from build123d import *

# Parameters (mm, degrees)
SKETCH1_W           = 177.8
SKETCH1_H           = 355.6
BOSS_EXTRUDE1_DEPTH = 12.7
BOSS_EXTRUDE2_DEPTH = 76.2


with BuildPart() as part:
    # Sketch1 → Boss-Extrude1 (new, symmetric)
    with BuildSketch(Plane(origin=(0, 0, 0), x_dir=(1, 0, 0), z_dir=(0, 1, 0))):
        Rectangle(SKETCH1_W, SKETCH1_H)
    extrude(amount=BOSS_EXTRUDE1_DEPTH, both=True)

    # Sketch2 → Boss-Extrude2 (add, symmetric)
    with BuildSketch(Plane(origin=(0, 0, 0), x_dir=(0, 0, -1), z_dir=(1, 0, 0))):
        with BuildLine():
            Line((-152.4, -12.7), (-152.4, 38.1))
            ThreePointArc((-152.4, 38.1), (-127, 63.5), (-101.6, 38.1))
            Line((-101.6, 38.1), (-101.6, -12.7))
            ThreePointArc((-101.6, -12.7), (-127, -38.1), (-152.4, -12.7))
        make_face()
        with BuildLine():
            Line((101.6, -12.7), (101.6, 38.1))
            ThreePointArc((101.6, 38.1), (127, 63.5), (152.4, 38.1))
            Line((152.4, 38.1), (152.4, -12.7))
            ThreePointArc((152.4, -12.7), (127, -38.1), (101.6, -12.7))
        make_face()
    extrude(amount=BOSS_EXTRUDE2_DEPTH, both=True)


solid = part.part
The model under review builds one solid part; all positions refer to its coordinate system, in mm. A direction names the side the tool comes from. Give positions to 0.01 mm unless a question says otherwise; leave off trailing zeros. Order: outer loops, then holes, each group sorted by start corner. A loop starts at its lowest first (then second) coordinate and runs counter-clockwise, first axis right, second up. Notation, with made-up numbers: M 12.5,-22.75 L 69.5,-22.75 A21 cw 69.5,8.25 Z; hole C 40.5,70.25 d8. An arc over 180 degrees is marked long. Use one line per item in the form item = value. Start each with the question number.
Item 1: We need section D-D on y = -31. Give the boundary of the cut face in (x, z), plus the area to 3 significant figures.
Item 2: The part is to be moulded in two halves that separate along Z. For faces 1 (the cylindrical face through (-1.067, -38.094, 126.441)), 2 (the flat face through (-76.2, -22, -127)), 3 (the flat face through (-1, 0, 177.8)), say which applies: pulls with the +Z half, pulls with the -Z half, needs draft (parallel to the pull), parting line crosses it, or undercut.
Item 3: Insertion check: pin 1 Ø7.5 at (x, y) = (-32, 25) entering from +Z; pin 2 Ø15 at (y, z) = (42.5, -117) entering from -X; pin 3 Ø12.5 at (y, z) = (-19.5, 120.5) entering from +X. Each pin has a flat end and moves straight along its axis. Give the tip position at first contact, or say it passes through.
Item 4: We need section A-A on y = 30.5. Give the boundary of the cut face in (x, z), plus the area to 3 significant figures.
Item 5: We need section C-C on z = -127. Give the boundary of the cut face in (x, y), plus the area to 3 significant figures.
Item 6: To check wall thickness, follow line 1 along Z through (x, y) = (-45, 16); line 2 along Y through (x, z) = (-9, 78.5); line 3 along Z through (x, y) = (47, 56.5). State the ranges of each line that lie inside material, in increasing order. Write a range as from..to.
Item 7: We need section B-B on x = 16. Give the boundary of the cut face in (y, z).
Item 8: For faces 4 (the flat face through (76.2, -22, 127)), 5 (the flat face through (-1, 26, 101.6)), 6 (the flat face through (76.2, 38, -127)), 7 (the flat face through (-1, 25, 152.4)), 8 (the flat face through (-76.2, 38, -127)), list the 3-axis set-ups (+Z, -Z, +X, -X, +Y, -Y) from which the entire face can be reached by the end or side of a thin tool; tool diameter is ignored.
Completed:
q1.outline = M -76.2,-144.61 L 76.2,-144.61 L 76.2,-109.39 L -76.2,-109.39 Z; M -76.2,109.39 L 76.2,109.39 L 76.2,144.61 L -76.2,144.61 Z
q1.area = 10,700 mm²
q2.face_1 = undercut
q2.face_2 = needs draft
q2.face_3 = pulls with the +Z half
q3.pin_1 = 152.4
q3.pin_2 = -76.2
q3.pin_3 = 76.2
q4.outline = M -76.2,-152.4 L 76.2,-152.4 L 76.2,-101.6 L -76.2,-101.6 Z; M -76.2,101.6 L 76.2,101.6 L 76.2,152.4 L -76.2,152.4 Z
q4.area = 15,500 mm²
q5.outline = M -88.9,-12.7 L -76.2,-12.7 L -76.2,-38.1 L 76.2,-38.1 L 76.2,-12.7 L 88.9,-12.7 L 88.9,12.7 L 76.2,12.7 L 76.2,63.5 L -76.2,63.5 L -76.2,12.7 L -88.9,12.7 Z
q5.area = 16,100 mm²
q6.line_1 = -152.4..-101.6, 101.6..152.4
q6.line_2 = -12.7..12.7
q6.line_3 = -144.51..-109.49, 109.49..144.51
q7.outline = M -12.7,-177.8 L 12.7,-177.8 L 12.7,-152.4 L 38.1,-152.4 A25.4 ccw 38.1,-101.6 L 12.7,-101.6 L 12.7,101.6 L 38.1,101.6 A25.4 ccw 38.1,152.4 L 12.7,152.4 L 12.7,177.8 L -12.7,177.8 L -12.7,152.4 A25.4 ccw -12.7,101.6 L -12.7,-101.6 A25.4 ccw -12.7,-152.4 Z
q8.face_4 = +Z, -Z, +X, -Y
q8.face_5 = +X, -X, +Y
q8.face_6 = +Z, -Z, +X, +Y
q8.face_7 = +Z, +X, -X, +Y
q8.face_8 = +Z, -Z, -X, +Y
